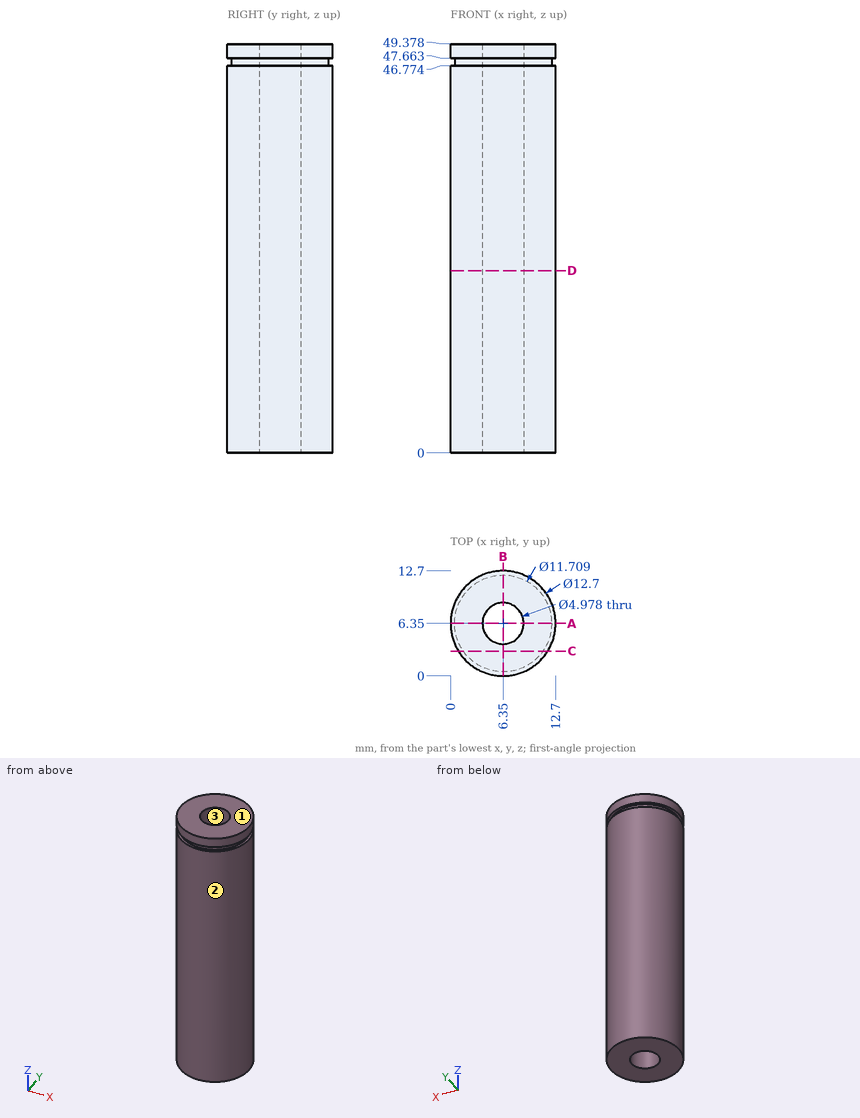
Here's the drawing with two shaded views (mm, measured from the low corner). I have some questions. Coordinates: 2 decimals unless noted, no trailing zeros. Order: outer loops, then holes, each group sorted by start corner. A loop starts at its lowest first (then second) coordinate and runs counter-clockwise, first axis right, second up. Notation, with made-up numbers: (36.5, -11) - (68.5, -11) arc R23 ccw to (68.5, 10) - close; hole circle Ø11 at (19.25, 36). An arc over 180 degrees is marked (long way). Use CSV: the item, a comma, the result in double quotes. Start each with the question number.
1. I'm going to push flat-ended pins straight in: pin 1 (2 mm diameter, centred on y = 1.5, z = 30.5, fed in from +X); pin 2 (6 mm diameter, centred on y = 3, z = 29, fed in from -X). Where does each tip first touch, or does it pass through?
2. Suppose I cut it at D-D on z = 22. List the corners of the cut face in (x, y) for me.
3. Suppose I cut it at C-C on y = 3. List the corners of the cut face in (x, z) for me (1 decimal), then the cut area to 3 significant figures.
4. Please list where these lines run through material, in increasing order: line 1 (Y direction, x = 6.35, z = 15.5); line 2 (Z direction, x = 0.5, y = 7.75); line 3 (X direction, y = 6.5, z = 33) (1 decimal). Write a range as from..to.
5. If we mould it in two halves opening along X, with no side actions, what happens to the marked faces 1, 2 and 3? For each: +X half, -X half, draft (parallel to the pull), parting line (faces both ways), or undercut.
6. Suppose I cut it at A-A on y = 6.35. List the corners of the cut face in (x, z) for me (1 decimal).
Output:
1,pin 1,"stops at x = 11.4"
1,pin 2,"stops at x = 0.01"
2,outline,"circle Ø12.7 at (6.35, 6.35); hole circle Ø4.98 at (6.35, 6.35)"
3,outline,"(1, 0) - (11.7, 0) - (11.7, 46.8) - (11.2, 46.8) - (11.2, 47.7) - (11.7, 47.7) - (11.7, 49.4) - (1, 49.4) - (1, 47.7) - (1.5, 47.7) - (1.5, 46.8) - (1, 46.8) - close"
3,area,"532 mm2"
4,line 1,"y = 0..3.86, 8.84..12.7"
4,line 2,"z = 0..46.77, 47.66..49.38"
4,line 3,"x = 0..3.9, 8.8..12.7"
5,face 1,"draft"
5,face 2,"parting line"
5,face 3,"undercut"
6,outline,"(0, 0) - (3.9, 0) - (3.9, 49.4) - (0, 49.4) - (0, 47.7) - (0.5, 47.7) - (0.5, 46.8) - (0, 46.8) - close; (8.8, 0) - (12.7, 0) - (12.7, 46.8) - (12.2, 46.8) - (12.2, 47.7) - (12.7, 47.7) - (12.7, 49.4) - (8.8, 49.4) - close"
